The model under review builds one solid part; all positions refer to its coordinate system, in mm. A direction names the side the tool comes from. Give positions to 0.01 mm unless a question says otherwise; leave off trailing zeros. Loops run counter-clockwise (first coordinate to the right, second up) from the corner with the lowest first, then second, coordinate; pieces in that order, holes last. Notation, with made-up numbers: (-35.5, -8.5) -> (1.5, -8.5) arc R17 cw to (1.5, -3.5) -> close; hole circle Ø11 at (-9.75, -30.75). An arc over 180 degrees is marked (long way). Write each question's results on one line, items separated by ' | '. Start each with the question number.
Q1. We need section D-D (z = 5.5). Write out the cut boundary in (x, y).
Q2. We need section A-A (z = 0). Write out the cut boundary in (x, y).
Q3. Wall thickness on L1, parallel to X at y = 20.5, z = 0; L2, parallel to Y at x = -3, z = 4; L3, parallel to X at y = 15, z = -0.25: over which ranges is each line inside the solid? List them lowest first. Write a range as [from, to].
Q4. We need section C-C (x = 35). Write out the cut boundary in (y, z).
Q5. We need section B-B (y = 5). Write out the cut boundary in (x, z), plus the area to 3 significant figures.
Q6. Mouldability with a two-part tool opening along Z and no side actions: class faces 1 (the face through (0, 11, -14.75)), 2 (the face through (0, 11, 14.75)), 3 (the face through (-48.496, 11.388, 0.324)), 4 (the face through (-28.555, 20.635, -0.846)) as released by +Z, released by -Z, zero draft, split by the parting line, or undercut.
Q7. Insertion check: pin 1 Ø1 at (y, z) = (13, 11.5) entering from +X; pin 2 Ø6 at (y, z) = (16.5, -4.5) entering from -X; pin 3 Ø5 at (y, z) = (7, -5) entering from -X. Each pin has a flat end and moves straight along its axis. Give the tip position at first contact, or say it passes through.
Q8. Machinability: for faces 5 (the face through (1, 23.1, -7)), 6 (the face through (41.445, 20.635, -0.846)), which of the approach directions +Z, -Z, +X, -X, +Y, -Y give a long, thin tool a straight path to every point of the face, cutting with its end or side? Answer none if there is none.
from build123d import *

# Parameters (mm, degrees)
BOSS_EXTRUDE1_DEPTH = 23.1
SKETCH2_R           = 6.5
CUT_EXTRUDE1_DEPTH  = 5


with BuildPart() as part:
    # Sketch1 → Boss-Extrude1 (new body)
    with BuildSketch(Plane(origin=(0, 0, 0), x_dir=(1, 0, 0), z_dir=(0, 1, 0))):
        with BuildLine():
            ThreePointArc((33.75, 14.75), (48.5, 0), (33.75, -14.75))
            Line((33.75, -14.75), (-33.75, -14.75))
            ThreePointArc((-33.75, -14.75), (-48.5, 0), (-33.75, 14.75))
            Line((-33.75, 14.75), (33.75, 14.75))
        make_face()
    extrude(amount=BOSS_EXTRUDE1_DEPTH)

    # Sketch2 → Cut-Extrude1 (cut)
    with BuildSketch(Plane(origin=(0, 23.1, 0), x_dir=(1, 0, 0), z_dir=(0, 1, 0))):
        with Locations(Location((0, 0, 0), (0, 0, 270))):
            Circle(SKETCH2_R)
        with Locations(Location((-35, 0, 0), (0, 0, 270))):
            Circle(SKETCH2_R)
        with Locations(Location((35, 0, 0), (0, 0, 270))):
            Circle(SKETCH2_R)
    extrude(amount=-CUT_EXTRUDE1_DEPTH, mode=Mode.SUBTRACT)


solid = part.part
Output:
1) outline: (-47.44, 0) -> (47.44, 0) -> (47.44, 23.1) -> (38.46, 23.1) -> (38.46, 18.1) -> (31.54, 18.1) -> (31.54, 23.1) -> (3.46, 23.1) -> (3.46, 18.1) -> (-3.46, 18.1) -> (-3.46, 23.1) -> (-31.54, 23.1) -> (-31.54, 18.1) -> (-38.46, 18.1) -> (-38.46, 23.1) -> (-47.44, 23.1) -> close
2) outline: (-48.5, 0) -> (48.5, 0) -> (48.5, 23.1) -> (41.5, 23.1) -> (41.5, 18.1) -> (28.5, 18.1) -> (28.5, 23.1) -> (6.5, 23.1) -> (6.5, 18.1) -> (-6.5, 18.1) -> (-6.5, 23.1) -> (-28.5, 23.1) -> (-28.5, 18.1) -> (-41.5, 18.1) -> (-41.5, 23.1) -> (-48.5, 23.1) -> close
3) L1: [-48.5, -41.5], [-28.5, -6.5], [6.5, 28.5], [41.5, 48.5] | L2: [0, 18.1] | L3: [-48.5, 48.5]
4) outline: (0, -14.7) -> (23.1, -14.7) -> (23.1, -6.5) -> (18.1, -6.5) -> (18.1, 6.5) -> (23.1, 6.5) -> (23.1, 14.7) -> (0, 14.7) -> close
5) outline: (-33.75, -14.75) -> (33.75, -14.75) arc R14.75 ccw to (33.75, 14.75) -> (-33.75, 14.75) arc R14.75 ccw to start | area: 2,670 mm2
6) face 1: released by -Z | face 2: released by +Z | face 3: split by the parting line | face 4: undercut
7) pin 1: x = 43.58 | pin 2: x = -48.42 | pin 3: x = -48.29
8) face 5: +Z, -Z, +X, -X, +Y | face 6: +Y
